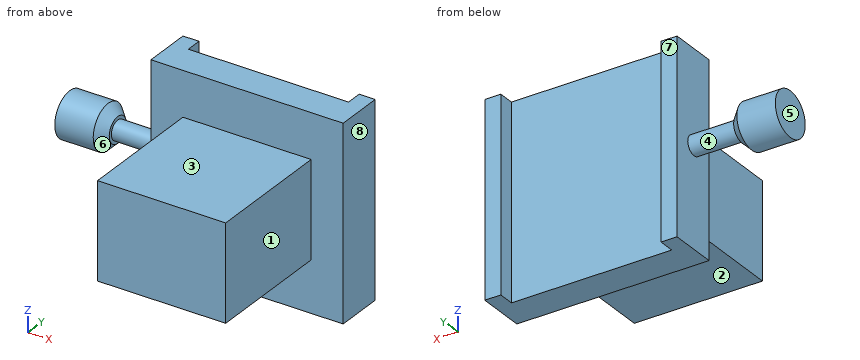
```python
from build123d import *

# Parameters (mm, degrees)
SKETCH1_W           = 40
SKETCH1_H           = 30
BOSS_EXTRUDE1_DEPTH = 40
BOSS_EXTRUDE2_DEPTH = 29
BOSS_EXTRUDE3_DEPTH = 31
BOSS_EXTRUDE4_START = -55
SKETCH4_R           = 3
BOSS_EXTRUDE4_DEPTH = 35
SKETCH5_R           = 7
BOSS_EXTRUDE5_DEPTH = 15
CHAMFER1_SIZE       = 3


with BuildPart() as part:
    # Sketch1 → Boss-Extrude1 (new body)
    with BuildSketch(Plane(origin=(0, 0, 0), x_dir=(1, 0, 0), z_dir=(0, 1, 0))):
        Rectangle(SKETCH1_W, SKETCH1_H)
    extrude(amount=-BOSS_EXTRUDE1_DEPTH)

    # Sketch3 → Boss-Extrude2 (add)
    with BuildSketch(Plane.XY):
        Polygon((25, 15), (30, 15), (30, 0), (-30, 0), (-30, 15), (-25, 15), (-25, 10), (25, 10), align=None)
    extrude(amount=BOSS_EXTRUDE2_DEPTH)

    # Sketch3<2> → Boss-Extrude3 (add)
    with BuildSketch(Plane.XY):
        Polygon((25, 15), (30, 15), (30, 0), (-30, 0), (-30, 15), (-25, 15), (-25, 10), (25, 10), align=None)
    extrude(amount=-BOSS_EXTRUDE3_DEPTH)

    # Sketch4 → Boss-Extrude4 (add)
    with BuildSketch(Plane(origin=(30, 0, 0), x_dir=(0, 0, -1), z_dir=(1, 0, 0)).offset(BOSS_EXTRUDE4_START)):
        with Locations((0, 7)):
            Circle(SKETCH4_R)
    extrude(amount=-BOSS_EXTRUDE4_DEPTH)

    # Sketch5 → Boss-Extrude5 (add)
    with BuildSketch(Plane.ZY.offset(60)):
        with Locations((0, 7)):
            Circle(SKETCH5_R)
    extrude(amount=-BOSS_EXTRUDE5_DEPTH)

    # Chamfer1
    chamfer1_edges = [part.edges().sort_by_distance(p)[0] for p in [
        (-45, 7, -7),
    ]]
    chamfer(chamfer1_edges, length=CHAMFER1_SIZE)


solid = part.part
```
Design review of the part built by this model. Coordinates are the model's own, in mm. Face numbers are marked on the shaded views. A direction names the side the tool comes from. Give positions to 0.01 mm unless a question says otherwise; leave off trailing zeros. Order: outer loops, then holes, each group sorted by start corner. A loop starts at its lowest first (then second) coordinate and runs counter-clockwise, first axis right, second up. Notation, with made-up numbers: M 44.5,-37.75 L 73.5,-37.75 A13 cw 73.5,-21.75 Z; hole C 44,29.5 d6. An arc over 180 degrees is marked long. One line per question, with ' | ' between items. Start each with the question number.
Q1. We need section D-D (z = -18). Write out the cut boundary in (x, y).
Q2. We need section C-C (x = 14). Write out the cut boundary in (y, z).
Q3. We need section A-A (z = -8). Write out the cut boundary in (x, y).
Q4. Machinability: for the marked faces 1, 2, 3 and 4, which of the approach directions +Z, -Z, +X, -X, +Y, -Y give a long, thin tool a straight path to every point of the face, cutting with its end or side? Answer none if there is none.
Q5. We need section B-B (y = 7). Write out the cut boundary in (x, z), plus the area to 3 significant figures.
Q6. For pin 1 Ø7.5 at (y, z) = (4, -13) entering from -X; pin 2 Ø1.5 at (y, z) = (13, 4.5) entering from -X; pin 3 Ø10 at (y, z) = (-30.5, 10) entering from -X; pin 4 Ø1.5 at (y, z) = (-20.5, 5) entering from +X, all flat-tipped, find the tip position at first contact; note any pin that passes through.
Q7. The part is to be moulded in two halves that separate along X. For the marked faces 5, 6, 7 and 8, say which applies: +X half, -X half, draft (parallel to the pull), parting line (faces both ways), or undercut.
Q8. For L1, parallel to Z at x = -5.5, y = -21.5; L2, parallel to Y at x = 18, z = -17; L3, parallel to X at y = -7, z = 4.5, list the stretches that pass through material, from the lowest coordinate up. Write a range as [from, to].
Returned:
1) outline: M -30,0 L 30,0 L 30,15 L 25,15 L 25,10 L -25,10 L -25,15 L -30,15 Z
2) outline: M -40,-15 L 0,-15 L 0,-31 L 10,-31 L 10,29 L 0,29 L 0,15 L -40,15 Z
3) outline: M -30,0 L -20,0 L -20,-40 L 20,-40 L 20,0 L 30,0 L 30,15 L 25,15 L 25,10 L -25,10 L -25,15 L -30,15 Z
4) face 1: +Z, -Z, +X, -Y | face 2: -Z, +X, -X, -Y | face 3: +Z, +X, -X, -Y | face 4: none
5) outline: M -60,-7 L -48,-7 L -45,-4 L -45,-3 L -30,-3 L -30,-31 L 30,-31 L 30,29 L -30,29 L -30,3 L -45,3 L -45,4 L -48,7 L -60,7 Z | area: 3,890 mm2
6) pin 1: x = -30 | pin 2: x = -60 | pin 3: x = -20 | pin 4: x = 20
7) face 5: -X half | face 6: undercut | face 7: draft | face 8: +X half
8) L1: [-15, 15] | L2: [0, 10] | L3: [-20, 20]
